Study the drawing (mm; zero at the part's minimum x, y, z) and answer. A direction names the side the tool comes from. Give positions to 0.01 mm unless a question says otherwise; leave off trailing zeros. Loops run counter-clockwise (first coordinate to the right, second up) from the corner with the lowest first, then second, coordinate; pieces in that order, holes last. Notation, with made-up numbers: M 53.5,86.25 L 104.5,86.25 A17 cw 104.5,108.25 Z; hole C 19.5,20 d8. An arc over 180 degrees is marked long. Return JSON: item names as keys, results as strings.
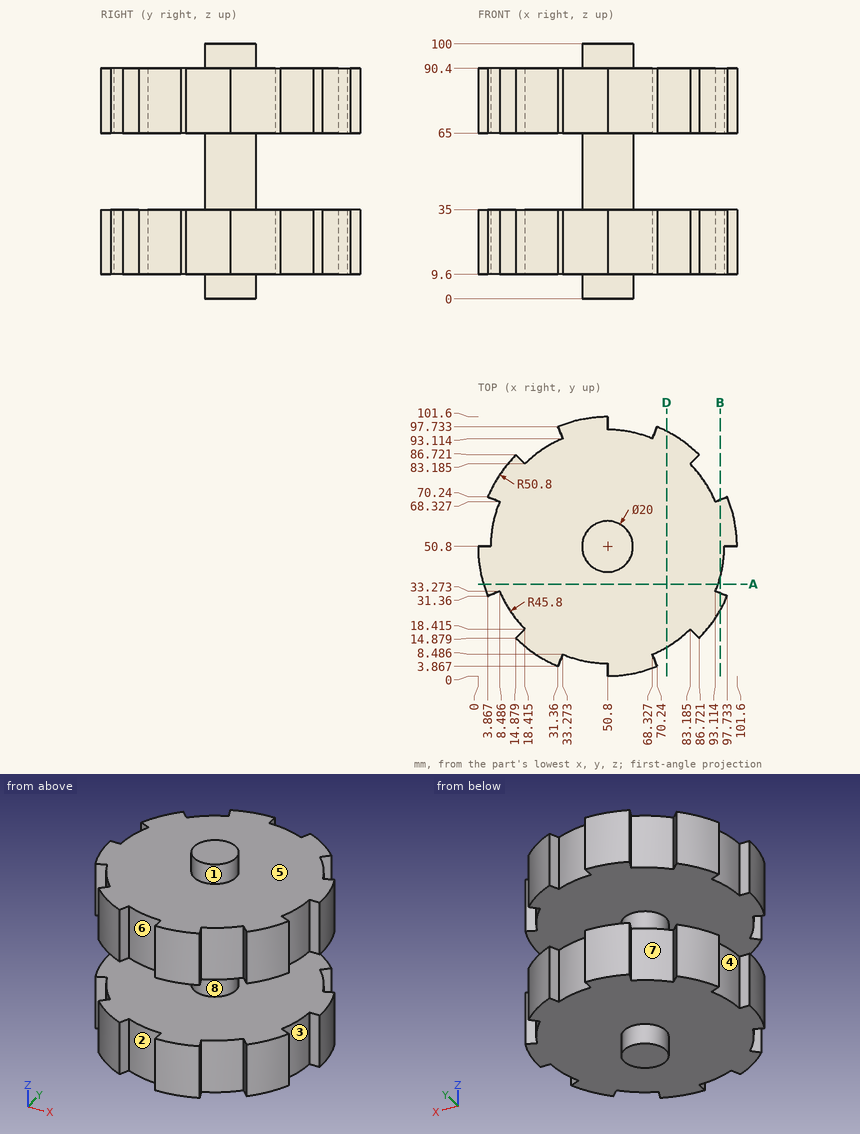
(1) Straight lines are drawn through the part: line 1 along Z through (x, y) = (26, 45); line 2 along Y through (x, z) = (17, 33.5) (1 decimal); line 3 along Y through (x, z) = (64, 30) (1 decimal). For each, find the intervals that lie inside material, in ascending order.
Values follow:
{"line 1": "9.6 to 35, 65 to 90.4", "line 2": "12.9 to 17, 19.9 to 84.6", "line 3": "1.7 to 94.7"}
(2) A tool of negligible diameter and unlimited length cuts with its end or side. For the marked faces 1, 2, 3 and 4, from which of +Z, -Z, +X, -X, +Y, -Y can it reach the whole face along a straight path? Write none if from no direction.
Values follow:
{"face 1": "+Z", "face 2": "+Z, -Z, -Y", "face 3": "+Z, -Z, +X", "face 4": "+Z, -Z, -X"}
(3) Determine the mould class of the marked faces 5, 6, 7 and 8 for opening direction X: released by +X, released by -X, zero draft, split by the parting line, or undercut.
Values follow:
{"face 5": "zero draft", "face 6": "undercut", "face 7": "undercut", "face 8": "split by the parting line"}
(4) The part is cut by section A-A (y = 36). Determine the outline of the cut face in (x, z).
Values follow:
{"outline": "M 2.2,9.6 L 94.14,9.6 L 94.14,35 L 2.2,35 Z; M 2.2,65 L 94.14,65 L 94.14,90.4 L 2.2,90.4 Z"}
(5) The part is cut by section B-B (x = 95). Determine the outline of the cut face in (y, z).
Values follow:
{"outline": "M 25.76,9.6 L 32.49,9.6 L 32.49,35 L 25.76,35 Z; M 25.76,65 L 32.49,65 L 32.49,90.4 L 25.76,90.4 Z; M 38.8,9.6 L 69.11,9.6 L 69.11,35 L 38.8,35 Z; M 38.8,65 L 69.11,65 L 69.11,90.4 L 38.8,90.4 Z"}
(6) The part is cut by section D-D (x = 74). Determine the outline of the cut face in (y, z), and give its area (3 significant figures).
Values follow:
{"outline": "M 11.31,9.6 L 95.99,9.6 L 95.99,35 L 11.31,35 Z; M 11.31,65 L 95.99,65 L 95.99,90.4 L 11.31,90.4 Z", "area": "4,300 mm²"}
(7) Given pin 1 (8 mm diameter, centred on y = 34, z = 48, fed in from -X); pin 2 (10 mm diameter, centred on x = 70, y = 63.5, fed in from +Z); pin 3 (8 mm diameter, centred on y = 30.5, z = 88.5, fed in from +X); pin 4 (4 mm diameter, centred on y = 1.5, z = 21, fed in from -X), each flat-ended and moving along its own axis, determine where each tip first touches the part or whether it passes through.
Values follow:
{"pin 1": "through", "pin 2": "z = 90.4", "pin 3": "x = 97.73", "pin 4": "x = 50.8"}
